CAD build for the part. Positions are in the model's coordinates, mm. Face numbers are marked on the shaded views. A direction names the side the tool comes from. Coordinates: 2 decimals unless noted, no trailing zeros. Loops run counter-clockwise (first coordinate to the right, second up) from the corner with the lowest first, then second, coordinate; pieces in that order, holes last.
1) Saw through at B-B, the plane y = -11. Write the cut outline in (x, z), and give its area (3 significant figures).
2) Wall check: line 1 along X through (y, z) = (-0.5, 2); line 2 along Y through (x, z) = (52, 14.5); line 3 along X through (y, z) = (5.5, 28). Give the ranges that are in metal, low to high.
3) Which spindle directions (+Z, -Z, +X, -X, +Y, -Y) get a long thin tool onto all of the face, cutting with end or side? Do the marked faces 1 and 2. Say none if no direction does.
4) Pin check, flat tips, straight feed: pin 1 Ø12 at (x, z) = (-21.5, 28) entering from -Y; pin 2 Ø11.5 at (x, z) = (37, 30.5) entering from -Y; pin 3 Ø5 at (x, y) = (9.5, 1) entering from +Z; pin 4 Ø7.5 at (x, y) = (51.5, 5.5) entering from -Z. Stop position of each tip, or through.
5) Saw through at C-C, the plane x = -9. Write the cut outline in (y, z).
6) Saw through at A-A, the plane x = 35. Write the cut outline in (y, z), and give its area (3 significant figures).
7) Two-plate mould, pull along X, no slides. Class the marked faces 3 and 4: +X half, -X half, draft (parallel to the pull), parting line (faces both ways), or undercut.
```python
from build123d import *

# Parameters (mm, degrees)
SKETCH_W          = 120
SKETCH_H          = 20
SKETCH_R          = 4
PAD_DEPTH         = 15
SKETCH001_W       = 40
SKETCH001_H       = 2
POCKET_DEPTH      = 265.600282
POCKET_DEPTH_BACK = 265.600282
SKETCH002_R       = 3.1
HOLE_DEPTH        = 20.001
POCKET001_DEPTH   = 5.5
PAD001_START      = -10
PAD001_DEPTH      = 5
SKETCH006_R       = 6.062178
POCKET002_DEPTH   = 10
POCKET003_DEPTH   = 273.798218
PAD002_START      = -20
PAD002_DEPTH      = 5
CHAMFER_SIZE      = 1
FILLET_R          = 4


with BuildPart() as part:
    # Sketch → Pad (new body, symmetric)
    with BuildSketch(Plane.XZ):
        with Locations((0, 10)):
            Rectangle(SKETCH_W, SKETCH_H)
        with Locations((-41, 10)):
            Circle(SKETCH_R, mode=Mode.SUBTRACT)
        with Locations((41, 10)):
            Circle(SKETCH_R, mode=Mode.SUBTRACT)
    extrude(amount=PAD_DEPTH, both=True)

    # Sketch001 → Pocket (cut, two sides)
    with BuildSketch(Plane.XZ) as pocket_sk:
        with Locations((-60, 10)):
            Rectangle(SKETCH001_W, SKETCH001_H)
    pocket = extrude(amount=-POCKET_DEPTH, mode=Mode.SUBTRACT) + extrude(pocket_sk.sketch, amount=POCKET_DEPTH_BACK, mode=Mode.SUBTRACT)

    # Mirrored: Pocket across Sketch001 V_Axis
    add(pocket.mirror(Plane(origin=(0, 0, 0), x_dir=(0, -1, 0), z_dir=(1, 0, 0))), mode=Mode.SUBTRACT)

    # Sketch002 → Hole (cut, through all)
    with BuildSketch(Plane.XY):
        with Locations((-52, 0)):
            Circle(SKETCH002_R)
        with Locations((52, 0)):
            Circle(SKETCH002_R)
    extrude(amount=HOLE_DEPTH, mode=Mode.SUBTRACT)

    # Sketch003 → Pocket001 (cut)
    with BuildSketch(Plane.XY):
        Polygon((-46.75, 3.031089), (-52, 6.062178), (-57.25, 3.031089), (-57.25, -3.031089), (-52, -6.062178), (-46.75, -3.031089), align=None)
    pocket001 = extrude(amount=POCKET001_DEPTH, mode=Mode.SUBTRACT)

    # Mirrored001: Pocket001 across Sketch003 V_Axis
    add(pocket001.mirror(Plane(origin=(0, 0, 0), x_dir=(0, 0, 1), z_dir=(1, 0, 0))), mode=Mode.SUBTRACT)

    # Sketch005 → Pad001 (join)
    with BuildSketch(Plane.XZ.offset(PAD001_START)):
        Polygon((0, 38), (-40, 38), (-45, 20), (0, 20), align=None)
    pad001 = extrude(amount=-PAD001_DEPTH)

    # Sketch006 → Pocket002 (cut)
    with BuildSketch(Plane.XZ):
        with Locations((-35, 20)):
            Circle(SKETCH006_R)
    pocket002 = extrude(amount=-POCKET002_DEPTH, mode=Mode.SUBTRACT)

    # Sketch004 → Pocket003 (cut, through all)
    with BuildSketch(Plane.XZ):
        with BuildLine():
            ThreePointArc((-31.5, 28), (-35, 31.5), (-38.5, 28))
            Line((-38.5, 28), (-38.5, 20))
            ThreePointArc((-38.5, 20), (-35, 16.5), (-31.5, 20))
            Line((-31.5, 28), (-31.5, 20))
        make_face()
    pocket003 = extrude(amount=-POCKET003_DEPTH, mode=Mode.SUBTRACT)

    # Sketch007 → Pad002 (join)
    with BuildSketch(Plane.YZ.offset(PAD002_START)):
        Polygon((10, 38), (6, 38), (0, 20), (10, 20), align=None)
    pad002 = extrude(amount=-PAD002_DEPTH)

    # Mirrored002: Pad002, Pad001, Pocket002, Pocket003 across YZ
    add(pad002.mirror(Plane.YZ))
    add(pad001.mirror(Plane.YZ))
    add(pocket002.mirror(Plane.YZ), mode=Mode.SUBTRACT)
    add(pocket003.mirror(Plane.YZ), mode=Mode.SUBTRACT)

    # Chamfer
    chamfer_edges = [part.edges().sort_by_distance(p)[0] for p in [
        (60, 0, 20),
        (60, 0, 0),
        (-60, 0, 20),
        (-60, 0, 0),
        (0, -15, 20),
        (0, -15, 0),
        (-60, -15, 15.5),
        (-60, -15, 4.5),
        (-60, 15, 4.5),
        (-60, 15, 15.5),
        (60, -15, 15.5),
        (60, -15, 4.5),
        (60, 15, 15.5),
        (60, 15, 4.5),
        (0, 15, 0),
    ]]
    chamfer(chamfer_edges, length=CHAMFER_SIZE)

    # Fillet
    fillet_edges = [part.edges().sort_by_distance(p)[0] for p in [
        (45, 12.5, 20),
        (40, 12.5, 38),
        (-40, 12.5, 38),
        (-45, 12.5, 20),
        (22.5, 6, 38),
        (-22.5, 6, 38),
    ]]
    fillet(fillet_edges, radius=FILLET_R)


solid = part.part
```
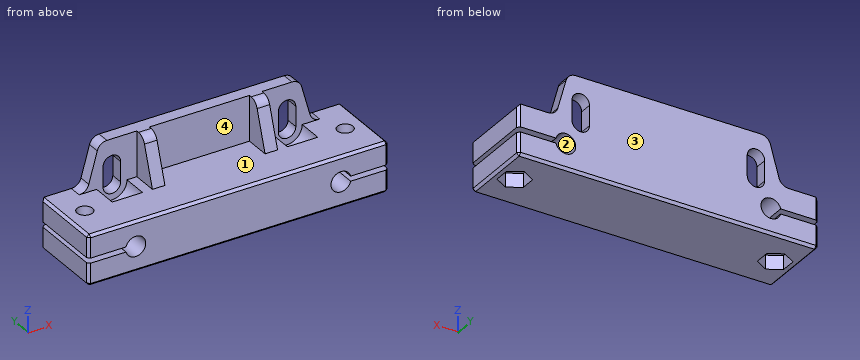
Data:
1. outline: (-60, 1) - (-59, 0) - (59, 0) - (60, 1) - (60, 9) - (44.87, 9) arc R4 cw (long way) to (44.87, 11) - (60, 11) - (60, 19) - (59, 20) - (-59, 20) - (-60, 19) - (-60, 11) - (-44.87, 11) arc R4 cw (long way) to (-44.87, 9) - (-60, 9) - close
1. area: 2,240 mm2
2. line 1: x = -60 to -57.25, -46.75 to 46.75, 57.25 to 60
2. line 2: y = -15 to -3.1, 3.1 to 15
2. line 3: x = -25 to -20, 20 to 25
3. face 1: +Z, -Y
3. face 2: +Y, -Y
4. pin 1: stops at y = 0.67
4. pin 2: stops at y = 10
4. pin 3: stops at z = 20
4. pin 4: stops at z = 0
5. outline: (-15, 1) - (-14, 0) - (14, 0) - (15, 1) - (15, 38) - (10, 38) - (10, 20) - (-14, 20) - (-15, 19) - close
6. outline: (-15, 1) - (-14, 0) - (14, 0) - (15, 1) - (15, 16.5) - (10, 16.5) - (10, 13.94) - (0, 13.94) - (0, 20) - (-14, 20) - (-15, 19) - close; (10, 31.5) - (15, 31.5) - (15, 38) - (10, 38) - close
6. area: 553 mm2
7. face 3: draft
7. face 4: undercut
